Model file for the job. Use its own axes, mm. Face numbers are marked on the shaded views. A direction names the side the tool comes from. Round coordinates to 2 decimals unless told otherwise and drop trailing zeros. Loops run counter-clockwise (first coordinate to the right, second up) from the corner with the lowest first, then second, coordinate; pieces in that order, holes last. Notation, with made-up numbers: M 71.5,58 L 108.5,58 A26 ccw 108.5,95 Z; hole C -26.75,-36.5 d3. An arc over 180 degrees is marked long. Use a Markdown table: item, result. Add a question column.
Q1. Cut at C-C (z = 25). Give the cut face in (x, y), plus the area to 3 significant figures.
Q2. Tool access for the marked faces 1 and 2: list every direction of +Z, -Z, +X, -X, +Y, -Y with a clear straight run to the whole face (end or side of a thin tool).
Q3. Cut at B-B (x = 0). State how many separate pieces and enclosed holes the cut face has, plus the area to 3 significant figures.
Q4. Cut at A-A (y = 0). Give the cut face in (x, z).
Q5. Mould opens along Y. For the marked faces 3, 4 and 5 say: +Y half, -Y half, draft (parallel to the pull), parting line (faces both ways), or undercut.
Q6. Pin check, flat tips, straight feed: pin 1 (8 mm diameter, centred on x = 7.5, z = 32, fed in from +Y); pin 2 (3 mm diameter, centred on y = -2.5, z = 31.5, fed in from -X); pin 3 (8 mm diameter, centred on x = 7, z = 9, fed in from +Y). Stop position of each tip, or through.
Q7. Cut at D-D (z = 35). Give the cut face in (x, y).
Q8. Probe line 1 (Y direction, x = 6.5, z = 28.5); line 2 (Y direction, x = -4.5, z = 9); line 3 (X direction, y = 19, z = 4). List the from-to ranges inside material, lowest first. Write a range as from..to.
Autodesk Inventor part; units mm, degrees
ref_plane "Work Plane1" through (0, 0, 0) normal (1, 0, 0) x (0, 1, 0)
ref_plane "Work Plane2" through (0, 0, 0) normal (0, 0, 1) x (1, 0, 0)
ref_plane "XZ Plane" through (0, 0, 0) normal (0, 1, 0) x (-1, 0, 0)
sketch "Sketch1" plane through (0, 0, 0) normal (0, 0, 1) x (1, 0, 0)
  circle A0 centre (0, 0) radius 22.5
  dimension "d0" = 45
extrude "Extrusion1" add sketch "Sketch1" along normal blind 8
ref_plane "Work Plane1" through (0, 0, 0) normal (1, 0, 0) x (0, 1, 0)
sketch "Sketch3" plane through (0, 0, 0) normal (1, 0, 0) x (0, 1, 0)
  line L0 (22.5, 8) -> (-22.5, 8)
  line L1 (22.5, 0) -> (-22.5, 0)
  line L2 (0, 8) -> (0, 41)
  line L3 (0, 41) -> (-13.5, 41)
  line L4 (-13.5, 41) -> (-15, 8)
  point P0 (0, 0)
  dimension "d4" = 27
  dimension "d5" = 33
  dimension "d6" = 30
revolve "Revolution1" add sketch "Sketch3" angle 360 about axis through (0, 0, 8) along (0, 0, 1)
fillet "Fillet1" radius 1.5 1 edges at (0, 15, 8)
sketch "Sketch5" plane through (0, 0, 0) normal (1, 0, 0) x (0, 1, 0)
  arc A0 (22.5, 0) -> (-22.5, 0) centre (0, -33.6749) ccw
  line L0 (22.5, 0) -> (-22.5, 0)
  point P0 (0, 0)
  dimension "d16" = 81
extrude "Extrusion2" cut sketch "Sketch5" along normal mid plane 45
fillet "Fillet2" radius 0.6 1 edges at (-22.5, 0, 8)
fillet "Fillet3" radius 1 1 edges at (0, 13.5, 41)
sketch "Sketch6" plane through (0, 0, 41) normal (0, 0, 1) x (1, 0, 0)
  circle A0 centre (0, 0) radius 13.5
hole "Hole2" at (0, 0, 41) direction (0, 0, -1) diameter 20 end through all counterbore diameter 22 counterbore depth 27
sketch "Sketch7" plane through (0, 0, 8) normal (0, 0, 1) x (1, 0, 0)
  point P0 (0, 0)
  point P1 (0, -19)
  point P2 (0, 19)
  dimension "d27" = 19
  dimension "d28" = 19
hole "Hole3" at (0, -19, 8) at (0, 19, 8) direction (0, 0, -1) diameter 3 end through all
ref_plane "Work Plane2" through (0, 0, 0) normal (0, 0, 1) x (1, 0, 0)
sketch "Sketch9" plane through (0, 0, 0) normal (0, 0, 1) x (1, 0, 0)
  circle A0 centre (0, 0) radius 22.5
  dimension "d39" = 45
properties part number "131" material "Aluminum 6061-AHC"
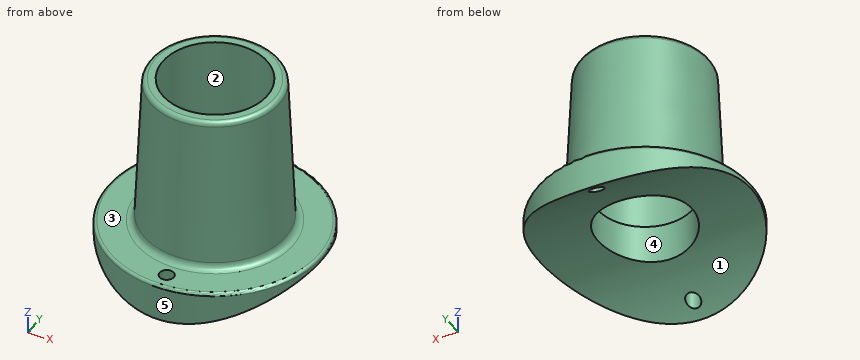
Checked values:
| question | item | result |
|---|---|---|
| 1 | outline | C 0,0 d28.45; hole C 0,0 d22 |
| 1 | area | 256 mm^2 |
| 2 | face 1 | -Z, +X, -X |
| 2 | face 2 | +Z |
| 3 | separate pieces | 4 |
| 3 | enclosed holes | 0 |
| 3 | area | 311 mm^2 |
| 4 | outline | M -22.5,6.83 L -10,6.83 L -10,14 L -11,14 L -11,41 L -12.54,41 A1 ccw -13.54,40.05 L -14.93,9.43 A1.5 cw -16.43,8 L -21.9,8 A0.6 ccw -22.5,7.4 Z; M 10,6.83 L 22.5,6.83 L 22.5,7.4 A0.6 ccw 21.9,8 L 16.43,8 A1.5 cw 14.93,9.43 L 13.54,40.05 A1 ccw 12.54,41 L 11,41 L 11,14 L 10,14 Z |
| 5 | face 3 | draft |
| 5 | face 4 | undercut |
| 5 | face 5 | parting line |
| 6 | pin 1 | stops at y = 13.48 |
| 6 | pin 2 | stops at x = -13.91 |
| 6 | pin 3 | stops at y = 22.25 |
| 7 | outline | C 0,0 d27.55; hole C 0,0 d22 |
| 8 | line 1 | y = -12.48..-8.87, 8.87..12.48 |
| 8 | line 2 | y = -14.33..-8.93, 8.93..14.33 |
| 8 | line 3 | x = -12.05..-1.5, 1.5..12.05 |
